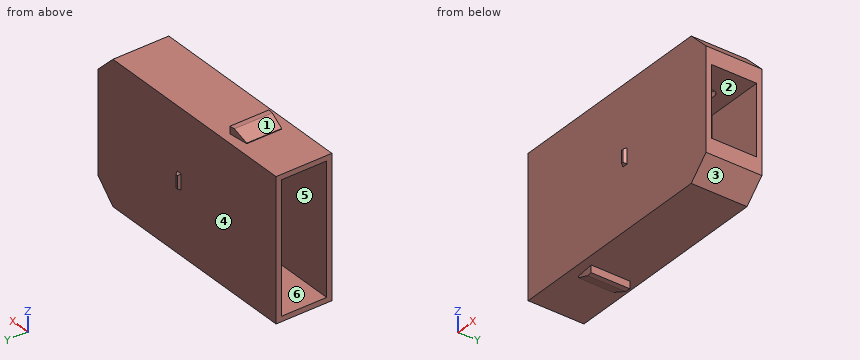
from build123d import *

# Parameters (mm, degrees)
SKETCH1_W           = 22.86
SKETCH1_H           = 13.716
BOSS_EXTRUDE1_DEPTH = 5.461
CHAMFER1_SIZE       = 1.905
SKETCH2_W           = 6.858
SKETCH2_H           = 4.445
CUT_EXTRUDE1_DEPTH  = 5.715
SHELL3_START        = 0.508
SHELL3_DEPTH        = 4.445
SKETCH3_R           = 1.27
CUT_EXTRUDE2_DEPTH  = 23.625255844
SKETCH4_W           = 0.508
SKETCH4_H           = 1.524
BOSS_EXTRUDE2_DEPTH = 0.254
BOSS_EXTRUDE2_TAPER = 30
SKETCH5_W           = 0.508
SKETCH5_H           = 1.524
BOSS_EXTRUDE3_DEPTH = 0.254
BOSS_EXTRUDE3_TAPER = 30
BOSS_EXTRUDE4_DEPTH = 0.7112
CUT_EXTRUDE3_DEPTH  = 28.511138389
BOSS_EXTRUDE6_DEPTH = 0.7112
CUT_EXTRUDE4_DEPTH  = 28.876190112
CUT_EXTRUDE5_REACH  = 28.223
SKETCH11_R          = 0.635
CUT_EXTRUDE6_DEPTH  = 24.12479948


# Read off the part's stored shape, not the designer's step: Shell3
with BuildPart() as part:
    # Sketch1 → Boss-Extrude1 (new body)
    with BuildSketch(Plane(origin=(0, 0, 0), x_dir=(1, 0, 0), z_dir=(0, 1, 0))):
        with Locations((-11.43, 6.858)):
            Rectangle(SKETCH1_W, SKETCH1_H)
    extrude(amount=BOSS_EXTRUDE1_DEPTH)

    # Chamfer1
    chamfer1_edges = [part.edges().sort_by_distance(p)[0] for p in [
        (0, 2.7305, 0),
        (0, 2.7305, -13.716),
    ]]
    chamfer(chamfer1_edges, length=CHAMFER1_SIZE)

    # Sketch2 → Cut-Extrude1 (cut)
    with BuildSketch(Plane(origin=(0, 0, 0), x_dir=(0, 0, -1), z_dir=(1, 0, 0))):
        with Locations((6.858, 2.7305)):
            Rectangle(SKETCH2_W, SKETCH2_H)
    extrude(amount=-CUT_EXTRUDE1_DEPTH, mode=Mode.SUBTRACT)

    # Shell3 outline → Shell3 (cut)
    with BuildSketch(Plane(origin=(0, 0, 0), x_dir=(1, 0, 0), z_dir=(0, 1, 0)).offset(SHELL3_START)):
        Polygon((-0.508, 2.11542049), (-0.508, 2.921), (-6.223, 2.921), (-6.223, 10.795), (-0.508, 10.795), (-0.508, 11.60057951), (-2.11542049, 13.208), (-22.86, 13.208), (-22.86, 0.508), (-2.11542049, 0.508), align=None)
    extrude(amount=SHELL3_DEPTH, mode=Mode.SUBTRACT)

    # Sketch3 → Cut-Extrude2 (cut, through all)
    with BuildSketch(Plane(origin=(-5.715, 0, 0), x_dir=(0, 0, -1), z_dir=(1, 0, 0))):
        with Locations((6.858, 2.7305)):
            Circle(SKETCH3_R)
    extrude(amount=-CUT_EXTRUDE2_DEPTH, mode=Mode.SUBTRACT)

    # Sketch4 → Boss-Extrude2 (add)
    with BuildSketch(Plane(origin=(0, 5.461, 0), x_dir=(1, 0, 0), z_dir=(0, 1, 0))):
        with Locations((-10.414, 6.858)):
            Rectangle(SKETCH4_W, SKETCH4_H)
    extrude(amount=BOSS_EXTRUDE2_DEPTH, taper=BOSS_EXTRUDE2_TAPER)

    # Sketch5 → Boss-Extrude3 (add)
    with BuildSketch(Plane.XZ):
        with Locations((-10.414, -6.858)):
            Rectangle(SKETCH5_W, SKETCH5_H)
    extrude(amount=BOSS_EXTRUDE3_DEPTH, taper=BOSS_EXTRUDE3_TAPER)

    # Sketch6 → Boss-Extrude4 (add)
    with BuildSketch(Plane.XY):
        Polygon((-15.8496, 0.8255), (-15.8496, 4.6355), (-17.7546, 4.445), (-17.7546, 1.016), align=None)
    extrude(amount=BOSS_EXTRUDE4_DEPTH)

    # Sketch7 → Cut-Extrude3 (cut, through all, along a direction that is not the sketch's normal)
    with BuildSketch(Plane(origin=(-0.075194059, -0.751940594, 0), x_dir=(-0.9950371902099893, 0.09950371902099862, 0), z_dir=(-0.09950371902099861, -0.9950371902099892, 0))):
        Polygon((17.767583076, -0.0508), (16.36108177, -0.7112), (17.767583076, -0.7112), align=None)
    extrude(amount=-CUT_EXTRUDE3_DEPTH, dir=(0, -1, 0), mode=Mode.SUBTRACT)

    # Sketch9 → Boss-Extrude6 (add)
    with BuildSketch(Plane(origin=(0, 0, -13.716), x_dir=(-1, 0, 0), z_dir=(0, 0, -1))):
        Polygon((17.7546, 1.016), (15.8496, 0.8255), (15.8496, 4.6355), (17.7546, 4.445), align=None)
    extrude(amount=BOSS_EXTRUDE6_DEPTH)

    # Sketch10 → Cut-Extrude4 (cut, through all, along a direction that is not the sketch's normal)
    with BuildSketch(Plane(origin=(-0.075194059, -0.751940594, 0), x_dir=(0.9950371902099892, -0.09950371902099901, 0), z_dir=(-0.09950371902099903, -0.9950371902099893, 0))):
        Polygon((-16.36108177, -14.4272), (-17.767583076, -13.843), (-17.767583076, -14.4272), align=None)
    extrude(amount=-CUT_EXTRUDE4_DEPTH, dir=(0, -1, 0), mode=Mode.SUBTRACT)

    # Cut-Extrude5: up to this face of the body (flat: up to its plane)
    cut_extrude5_end = Plane(part.part.faces().sort_by_distance((-12.487710245, 2.7305, -13.208))[0])
    # Sketch11 → Cut-Extrude5 (cut, up to the picked face)
    with BuildSketch(Plane.XY.offset(-2.921), mode=Mode.PRIVATE) as cut_extrude5_sk1:
        with Locations(Location((-3.461534283, 2.805193331, 0), (0, 0, 180))):
            Circle(SKETCH11_R)
    cut_extrude5_tool1 = split(extrude(cut_extrude5_sk1.sketch, amount=-CUT_EXTRUDE5_REACH, mode=Mode.PRIVATE), bisect_by=cut_extrude5_end, keep=Keep.BOTH, mode=Mode.PRIVATE)
    add(cut_extrude5_tool1.solids().sort_by(Axis((-3.461534, 2.805193, -2.921), (0, 0, -1)))[0], mode=Mode.SUBTRACT)

    # Sketch12 → Cut-Extrude6 (cut, through all)
    with BuildSketch(Plane(origin=(-5.715, 0, 0), x_dir=(0, 0, -1), z_dir=(1, 0, 0))):
        with BuildLine():
            Line((5.969, 3.63746141), (5.969, 4.295230705))
            Line((5.969, 4.295230705), (7.747, 4.295230705))
            Line((7.747, 4.295230705), (7.747, 3.63746141))
            ThreePointArc((7.747, 3.63746141), (6.858, 4.0005), (5.969, 3.63746141))
        make_face()
        with BuildLine():
            Line((5.969, 1.82353859), (5.969, 1.165769295))
            Line((5.969, 1.165769295), (7.747, 1.165769295))
            Line((7.747, 1.165769295), (7.747, 1.82353859))
            ThreePointArc((7.747, 1.82353859), (6.858, 1.4605), (5.969, 1.82353859))
        make_face()
    extrude(amount=-CUT_EXTRUDE6_DEPTH, mode=Mode.SUBTRACT)


solid = part.part
Could you check a few things on this model? Use its own coordinates, in mm. Face numbers are marked on the shaded views. A direction names the side the tool comes from. Coordinates: 2 decimals unless noted, no trailing zeros. Loops run counter-clockwise (first coordinate to the right, second up) from the corner with the lowest first, then second, coordinate; pieces in that order, holes last.
1. For P1, Ø2, axis at x = -4, y = 2, coming from the -Z side; P2, Ø1, axis at x = -18, z = -4.5, coming from the +Y side; P3, Ø1.3, axis at x = -3.5, y = 4, coming from the +Z side, each with a flat end and sliding along its axis, tell me the tip position at first contact or that it passes through.
2. For the marked faces 1 and 2, which set-ups out of +Z, -Z, +X, -X, +Y, -Y let a thin tool reach every point of the face, with its end or its side?
3. Imagine slicing it at B-B (z = -9.25). Please give me the cut outline in (x, y) (3 decimals), and give its area (3 significant figures).
4. Imagine slicing it at A-A (x = -9). Please give me the cut outline in (y, z), and give its area (3 significant figures).
5. Imagine slicing it at C-C (x = -3.25). Please give me the cut outline in (y, z) (3 decimals), and give its area (3 significant figures).
6. Imagine slicing it at D-D (y = 3.05). Give the number of separate pieces and of enclosed holes in the cut face, and give its area (3 significant figures).
7. I need wall thicknesses on L1, parallel to Z at x = -6, y = 2.75 (3 decimals); L2, parallel to Z at x = -5.25, y = 3.15 (3 decimals); L3, parallel to Z at x = -18.75, y = 1.2. Which ranges of each line are inside material? Lowest first, please.
8. We'd pull the mould along Z, two halves only. Please class the marked faces 3, 4, 5 and 6: released by +Z, released by -Z, zero draft, split by the parting line, or undercut.
Computed values:
1. P1: stops at z = -13.72
1. P2: stops at y = 5.46
1. P3: stops at z = 0
2. face 1: +Z, -X, +Y, -Y
2. face 2: +X
3. outline: (-22.86, 0) - (0, 0) - (0, 0.508) - (-5.715, 0.508) - (-5.715, 4.953) - (0, 4.953) - (0, 5.461) - (-22.86, 5.461) - (-22.86, 4.953) - (-6.223, 4.953) - (-6.223, 0.508) - (-22.86, 0.508) - close
3. area: 25.5 mm2
4. outline: (0, -13.72) - (5.46, -13.72) - (5.46, 0) - (0, 0) - close; hole (0.51, -13.21) - (4.95, -13.21) - (4.95, -0.51) - (0.51, -0.51) - close
4. area: 18.5 mm2
5. outline: (0, -13.716) - (5.461, -13.716) - (5.461, 0) - (0, 0) - close; hole (0.508, -13.208) - (4.953, -13.208) - (4.953, -10.795) - (3.404, -10.795) - (3.404, -10.287) - (4.953, -10.287) - (4.953, -3.429) - (3.404, -3.429) - (3.404, -2.921) - (4.953, -2.921) - (4.953, -0.508) - (0.508, -0.508) - (0.508, -2.921) - (2.206, -2.921) - (2.206, -3.429) - (0.508, -3.429) - (0.508, -10.287) - (2.206, -10.287) - (2.206, -10.795) - (0.508, -10.795) - close
5. area: 21.8 mm2
6. separate pieces: 4
6. enclosed holes: 0
6. area: 33.8 mm2
7. L1: z = -13.716 to -13.208, -10.795 to -8.128, -5.588 to -2.921, -0.508 to 0
7. L2: z = -13.716 to -13.208, -10.795 to -10.287, -3.429 to -2.921, -0.508 to 0
7. L3: z = -13.72 to -13.21, -0.51 to 0
8. face 3: released by -Z
8. face 4: zero draft
8. face 5: undercut
8. face 6: undercut
